Check sheet for the modelled part. Datum: model origin and axes. Units: mm. A direction names the side the tool comes from. Round coordinates to 2 decimals unless told otherwise and drop trailing zeros. Order: outer loops, then holes, each group sorted by start corner. A loop starts at its lowest first (then second) coordinate and runs counter-clockwise, first axis right, second up.
```python
from build123d import *

# Parameters (mm, degrees)
SKETCH2_R           = 4.5
BOSS_EXTRUDE1_DEPTH = 5
BOSS_EXTRUDE4_DEPTH = 31
BOSS_EXTRUDE5_DEPTH = 31
BOSS_EXTRUDE6_DEPTH = 31
SKETCH5_W           = 2.05
SKETCH5_H           = 17
BOSS_EXTRUDE7_DEPTH = 15.25
CUT_EXTRUDE3_DEPTH  = 5
CUT_EXTRUDE4_DEPTH  = 15
FILLET2_R           = 4
SKETCH8_R           = 1.75
CUT_EXTRUDE5_DEPTH  = 10
SKETCH8_3_R         = 11.5
SKETCH8_3_R_2       = 4.5
CUT_EXTRUDE6_DEPTH  = 3.5
BOSS_EXTRUDE8_DEPTH = 31


with BuildPart() as part:
    # Sketch2 → Boss-Extrude1 (new body)
    with BuildSketch(Plane(origin=(0, 0, 0), x_dir=(1, 0, 0), z_dir=(0, 1, 0))):
        with BuildLine():
            Line((30.852324511, 42.360372936), (0, 26))
            ThreePointArc((0, 26), (-26, 0), (0, -26))
            Line((0, -26), (30.852324511, -42.360372936))
            ThreePointArc((30.852324511, -42.360372936), (109.945, 0), (30.852324511, 42.360372936))
        make_face()
        Circle(SKETCH2_R, mode=Mode.SUBTRACT)
        with Locations((59.055, 0)):
            Circle(SKETCH2_R, mode=Mode.SUBTRACT)
    extrude(amount=BOSS_EXTRUDE1_DEPTH)

    # Sketch3 → Boss-Extrude4 (add)
    with BuildSketch(Plane(origin=(0, 5, 0), x_dir=(1, 0, 0), z_dir=(0, 1, 0))):
        with BuildLine():
            Line((30.852324511, 42.360372936), (0, 26))
            ThreePointArc((0, 26), (-26, 0), (0, -26))
            Line((0, -26), (30.852324511, -42.360372936))
            ThreePointArc((30.852324511, -42.360372936), (109.945, 0), (30.852324511, 42.360372936))
        make_face()
        with BuildLine():
            ThreePointArc((0, -21), (-21, 0), (0, 21))
            Line((0, 21), (35.989825914, 40.084687562))
            ThreePointArc((35.989825914, 40.084687562), (71.67744287, 44.491104375), (99.734041687, 22))
            Line((99.734041687, 22), (102, 22))
            Line((102, 22), (102, 17.161334667))
            ThreePointArc((102, 17.161334667), (105.301993768, 0), (102, -17.161334667))
            Line((102, -17.161334667), (102, -22))
            Line((102, -22), (99.734041687, -22))
            ThreePointArc((99.734041687, -22), (71.67744287, -44.491104375), (35.989825914, -40.084687562))
            Line((35.989825914, -40.084687562), (0, -21))
        make_face(mode=Mode.SUBTRACT)
    extrude(amount=BOSS_EXTRUDE4_DEPTH)

    # Sketch3<10> → Boss-Extrude5 (add)
    with BuildSketch(Plane(origin=(0, 5, 0), x_dir=(1, 0, 0), z_dir=(0, 1, 0))):
        with BuildLine():
            Line((102, 22), (99.734041687, 22))
            ThreePointArc((99.734041687, 22), (100.936956229, 19.613418238), (102, 17.161334667))
            Line((102, 17.161334667), (102, 22))
        make_face()
        with BuildLine():
            ThreePointArc((102, -17.161334667), (100.936956229, -19.613418238), (99.734041687, -22))
            Line((99.734041687, -22), (102, -22))
            Line((102, -22), (102, -17.161334667))
        make_face()
    extrude(amount=BOSS_EXTRUDE5_DEPTH)

    # Sketch2<6> → Boss-Extrude6 (add)
    with BuildSketch(Plane(origin=(0, 0, 0), x_dir=(1, 0, 0), z_dir=(0, 1, 0))):
        with BuildLine():
            Line((127.435, 8.5), (109.23011435, 8.5))
            ThreePointArc((109.23011435, 8.5), (109.351284572, 7.750861777), (109.461270443, 7))
            Line((109.461270443, 7), (125.385, 7))
            Line((125.385, 7), (125.385, 0))
            Line((125.385, 0), (127.435, 0))
            Line((127.435, 0), (127.435, 8.5))
        make_face()
        with BuildLine():
            Line((127.435, -8.5), (127.435, 0))
            Line((127.435, 0), (125.385, 0))
            Line((125.385, 0), (125.385, -7))
            Line((125.385, -7), (109.461270443, -7))
            ThreePointArc((109.461270443, -7), (109.351284572, -7.750861777), (109.23011435, -8.5))
            Line((109.23011435, -8.5), (127.435, -8.5))
        make_face()
    extrude(amount=BOSS_EXTRUDE6_DEPTH)

    # Sketch5 → Boss-Extrude7 (add)
    with BuildSketch(Plane(origin=(0, 31, 0), x_dir=(1, 0, 0), z_dir=(0, 1, 0))):
        with Locations((126.41, 0)):
            Rectangle(SKETCH5_W, SKETCH5_H)
    extrude(amount=BOSS_EXTRUDE7_DEPTH)

    # Sketch6 → Cut-Extrude3 (cut)
    with BuildSketch(Plane(origin=(127.435, 0, 0), x_dir=(0, 0, -1), z_dir=(1, 0, 0))):
        with BuildLine():
            ThreePointArc((1.25, 43), (0.883883476, 43.883883476), (0, 44.25))
            Line((0, 44.25), (0, 41.75))
            ThreePointArc((0, 41.75), (0.883883476, 42.116116524), (1.25, 43))
        make_face()
        with BuildLine():
            Line((0, 41.75), (0, 44.25))
            ThreePointArc((0, 44.25), (-1.25, 43), (0, 41.75))
        make_face()
        with BuildLine():
            ThreePointArc((1.25, 33.5), (0.883883476, 34.383883476), (0, 34.75))
            Line((0, 34.75), (0, 32.25))
            ThreePointArc((0, 32.25), (0.883883476, 32.616116524), (1.25, 33.5))
        make_face()
        with BuildLine():
            Line((0, 32.25), (0, 34.75))
            ThreePointArc((0, 34.75), (-1.25, 33.5), (0, 32.25))
        make_face()
    extrude(amount=-CUT_EXTRUDE3_DEPTH, mode=Mode.SUBTRACT)

    # Sketch2<7> → Cut-Extrude4 (cut)
    with BuildSketch(Plane(origin=(0, 0, 0), x_dir=(1, 0, 0), z_dir=(0, 1, 0))):
        with BuildLine():
            Line((127.435, -8.5), (127.435, 0))
            Line((127.435, 0), (125.385, 0))
            Line((125.385, 0), (125.385, -7))
            Line((125.385, -7), (109.461270443, -7))
            ThreePointArc((109.461270443, -7), (109.351284572, -7.750861777), (109.23011435, -8.5))
            Line((109.23011435, -8.5), (127.435, -8.5))
        make_face()
        with BuildLine():
            Line((127.435, 8.5), (109.23011435, 8.5))
            ThreePointArc((109.23011435, 8.5), (109.351284572, 7.750861777), (109.461270443, 7))
            Line((109.461270443, 7), (125.385, 7))
            Line((125.385, 7), (125.385, 0))
            Line((125.385, 0), (127.435, 0))
            Line((127.435, 0), (127.435, 8.5))
        make_face()
    extrude(amount=CUT_EXTRUDE4_DEPTH, mode=Mode.SUBTRACT)

    # Fillet2
    fillet2_edges = [part.edges().sort_by_distance(p)[0] for p in [
        (125.385, 31, 7.75),
        (125.385, 31, -7.75),
        (126.41, 46.25, -8.5),
        (126.41, 46.25, 8.5),
        (109.351284572, 31, -7.750861777),
        (109.23011435, 23, -8.5),
        (109.351284572, 31, 7.750861777),
        (109.23011435, 23, 8.5),
    ]]
    fillet(fillet2_edges, radius=FILLET2_R)

    # Sketch8 → Cut-Extrude5 (cut)
    with BuildSketch(Plane.XZ):
        with Locations((0, 14)):
            Circle(SKETCH8_R)
        with Locations((14, 0)):
            Circle(SKETCH8_R)
        with Locations((0, -14)):
            Circle(SKETCH8_R)
        with Locations((-14, 0)):
            Circle(SKETCH8_R)
    extrude(amount=-CUT_EXTRUDE5_DEPTH, mode=Mode.SUBTRACT)

    # Sketch8<3> → Cut-Extrude6 (cut)
    with BuildSketch(Plane.XZ):
        Circle(SKETCH8_3_R)
        Circle(SKETCH8_3_R_2, mode=Mode.SUBTRACT)
    extrude(amount=-CUT_EXTRUDE6_DEPTH, mode=Mode.SUBTRACT)

    # Sketch3<13> → Boss-Extrude8 (add)
    with BuildSketch(Plane(origin=(0, 5, 0), x_dir=(1, 0, 0), z_dir=(0, 1, 0))):
        with BuildLine():
            ThreePointArc((24.5, -12.260820261), (23.824264635, -9.889112016), (22, -8.229691387))
            Line((22, -8.229691387), (22, -16.291949135))
            ThreePointArc((22, -16.291949135), (23.824264635, -14.632528506), (24.5, -12.260820261))
        make_face()
        with BuildLine():
            Line((22, -16.291949135), (22, -8.229691387))
            ThreePointArc((22, -8.229691387), (15.5, -12.260820261), (22, -16.291949135))
        make_face()
    extrude(amount=BOSS_EXTRUDE8_DEPTH)


solid = part.part
```
Item 1: Release check for a two-part mould opening along Z. For faces 5 (the cylindrical face through (126.424, 45.109, 7.297)), 6 (the cylindrical face through (-1.5, 1.7, 11.4)), 7 (the flat face through (41, 0, -1)), 8 (the flat face through (117, 23, -7)) record: released by +Z, released by -Z, zero draft, split by the parting line, or undercut.
Answer:
face 5: released by +Z
face 6: undercut
face 7: zero draft
face 8: undercut
Item 2: Access from +Z, -Z, +X, -X, +Y, -Y to the whole of each face (thin tool, end or side, straight path). Record for faces 1 (the flat face through (120, 22, -8.5)), 2 (the cylindrical face through (-21, 20, 0)), 3 (the cylindrical face through (124.24, 32.2, -7.76)), 4 (the flat face through (118, 23, 7)).
Answer:
face 1: -Z, +X, +Y, -Y
face 2: +Y
face 3: +Z, -Z, +Y
face 4: +Y, -Y
Item 3: Sectioned sample at B-B (x = 117). Record the cut outline in (y, z), and give its area (3 significant figures).
Answer:
outline: (15, -8.5) - (31, -8.5) - (31, -7) - (15, -7) - close; (15, 7) - (31, 7) - (31, 8.5) - (15, 8.5) - close
area: 48.0 mm2
Item 4: Sectioned sample at A-A (y = 17). Record the cut outline in (x, z) (3 decimals).
Answer:
outline: (0, -26) - (30.852, -42.36) arc R50.89 ccw to (108.608, -11.589) arc R4 cw to (112.503, -8.5) - (127.435, -8.5) - (127.435, 8.5) - (112.503, 8.5) arc R4 cw to (108.608, 11.589) arc R50.89 ccw to (30.852, 42.36) - (0, 26) arc R26 ccw to start; circle Ø9 at (20, 12.261); hole (0, -21) - (35.99, -40.085) arc R46.247 ccw (long way) to (35.99, 40.085) - (0, 21) arc R21 ccw to start; hole (109.461, -7) - (125.385, -7) - (125.385, 7) - (109.461, 7) arc R50.89 cw to start
Item 5: Sectioned sample at C-C (z = 14). Record the cut outline in (x, y).
Answer:
outline: (-21.91, 0) - (-1.75, 0) - (-1.75, 5) - (-15.65, 5) - (-15.65, 36) - (-21.91, 36) - close; (1.75, 0) - (107.98, 0) - (107.98, 36) - (103.13, 36) - (103.13, 5) - (24.15, 5) - (24.15, 36) - (15.85, 36) - (15.85, 5) - (1.75, 5) - close
Item 6: Sectioned sample at D-D (x = 43.5). Record the cut outline in (y, z).
Answer:
outline: (0, -48.45) - (36, -48.45) - (36, -43.55) - (5, -43.55) - (5, 43.55) - (36, 43.55) - (36, 48.45) - (0, 48.45) - close
Item 7: Go/stop test with flat-tipped pins: P1, Ø11.5, axis at x = -5.5, z = -0.5, coming from the -Y side; P2, Ø11.5, axis at x = 59.055, z = 0, coming from the +Y side; P3, Ø0.5, axis at x = 117.5, z = -7.5, coming from the +Y side. Record where each tip stops, or that it passes through.
Answer:
P1: stops at y = 3.5
P2: stops at y = 5
P3: stops at y = 31
Item 8: Scan lines: line 1 along Z through (x, y) = (0, 1.7); line 2 along X through (y, z) = (5.5, 15.5); line 3 along Z through (x, y) = (21, 18). Record each from-to range of solid material in increasing order.
Answer:
line 1: z = -26 to -15.75, -12.25 to -11.5, 11.5 to 12.25, 15.75 to 26
line 2: x = -20.87 to -14.17, 16.88 to 23.12, 102.63 to 107.53
line 3: z = -37.14 to -32.14, 7.87 to 16.65, 32.14 to 37.14
